Model file for the job. Use its own axes, mm. A direction names the side the tool comes from. Coordinates: 2 decimals unless noted, no trailing zeros. Order: outer loops, then holes, each group sorted by start corner. A loop starts at its lowest first (then second) coordinate and runs counter-clockwise, first axis right, second up. Notation, with made-up numbers: M 39.25,-9.75 L 88.25,-9.75 A14 cw 88.25,11.25 Z; hole C -21,33 d7. An arc over 180 degrees is marked long. Return JSON: item names as keys, results as strings.
```python
from build123d import *

# Parameters (mm, degrees)
BOSS_EXTRUDE1_DEPTH = 10
SKETCH2_W           = 30
SKETCH2_H           = 20
SKETCH2_W_2         = 20
SKETCH2_H_2         = 10
BOSS_EXTRUDE2_DEPTH = 5


with BuildPart() as part:
    # Sketch1 → Boss-Extrude1 (new body)
    with BuildSketch(Plane.XY):
        with BuildLine():
            Line((-75, 0), (-55, 0))
            ThreePointArc((-55, 0), (-4.793565851, 54.790708395), (54.164426416, 9.550649772))
            Line((54.164426416, 9.550649772), (73.860581476, 13.023613325))
            ThreePointArc((73.860581476, 13.023613325), (-6.536680706, 74.714602357), (-75, 0))
        make_face()
    extrude(amount=BOSS_EXTRUDE1_DEPTH)

    # Sketch2 → Boss-Extrude2 (add)
    with BuildSketch(Plane.XZ):
        with Locations((-65, 5)):
            Rectangle(SKETCH2_W, SKETCH2_H)
        with Locations((-65, 5)):
            Rectangle(SKETCH2_W_2, SKETCH2_H_2, mode=Mode.SUBTRACT)
        Polygon((-65, 5), (-75, 10), (-75, 0), align=None)
        Polygon((-55, 10), (-75, 10), (-65, 5), align=None)
        Polygon((-55, 10), (-65, 5), (-55, 0), align=None)
        Polygon((-55, 0), (-65, 5), (-75, 0), align=None)
    extrude(amount=BOSS_EXTRUDE2_DEPTH)


solid = part.part
```
Item 1: Wall check: line 1 (X direction, y = 39, z = 3.5); line 2 (Z direction, x = -37, y = 47); line 3 (X direction, y = 20.5, z = 7.5). Give the ranges that are in metal, low to high.
Check result:
{"line 1": "x = -64.06 to -38.78, 38.78 to 64.06", "line 2": "z = 0 to 10", "line 3": "x = -72.14 to -51.04, 51.04 to 72.14"}
Item 2: Saw through at C-C (x = -63.5). Write the cut outline in (y, z).
Check result:
{"outline": "M -5,-5 L 0,-5 L 0,0 L 39.91,0 L 39.91,10 L 0,10 L 0,15 L -5,15 Z"}
Item 3: 3-axis set-ups, long thin cutter, end or side, ignore diameter. For faces 1 (the flat face through (-18, 55, 10)), 2 (the flat face through (-18, 55, 0)), 3 (the flat face through (-50, -2, 5)): which of +Z, -Z, +X, -X, +Y, -Y reach the whole face in a straight line?
Check result:
{"face 1": "+Z, +X, -X, +Y", "face 2": "-Z, +X, -X, +Y", "face 3": "+Z, -Z, +X, -Y"}
Item 4: Saw through at D-D (y = 49). Write the cut outline in (x, z), and give its area (3 significant figures).
Check result:
{"outline": "M -56.78,0 L -24.98,0 L -24.98,10 L -56.78,10 Z; M 24.98,0 L 56.78,0 L 56.78,10 L 24.98,10 Z", "area": "636 mm2"}
Item 5: Drop flat-ended pins along their axis: pin 1 Ø8 at (x, z) = (15, 5.5) entering from -Y; pin 2 Ø3 at (x, y) = (6, 53) entering from +Z; pin 3 Ø3 at (x, y) = (53, 53) entering from -Z; pin 4 Ø1.5 at (y, z) = (-2, 0) entering from +X. Give the stop position or say it passes through.
Check result:
{"pin 1": "stops at y = 51.61", "pin 2": "passes through", "pin 3": "stops at z = 0", "pin 4": "stops at x = -50"}
Item 6: Saw through at A-A (y = 36). Write the cut outline in (x, z).
Check result:
{"outline": "M -65.8,0 L -41.58,0 L -41.58,10 L -65.8,10 Z; M 41.58,0 L 65.8,0 L 65.8,10 L 41.58,10 Z"}
Item 7: Saw through at B-B (z = 2.25). Write the cut outline in (x, y).
Check result:
{"outline": "M -80,-5 L -50,-5 L -50,0 L -55,0 A55 cw 54.16,9.55 L 73.86,13.02 A75 ccw -75,0 L -80,0 Z"}
